Design review of the part shown in the three views and the two pictorial views. Dimensions are in mm from the part's minimum x, y and z. Round coordinates to 2 decimals unless told otherwise and drop trailing zeros. Order: outer loops, then holes, each group sorted by start corner. A loop starts at its lowest first (then second) coordinate and runs counter-clockwise, first axis right, second up.
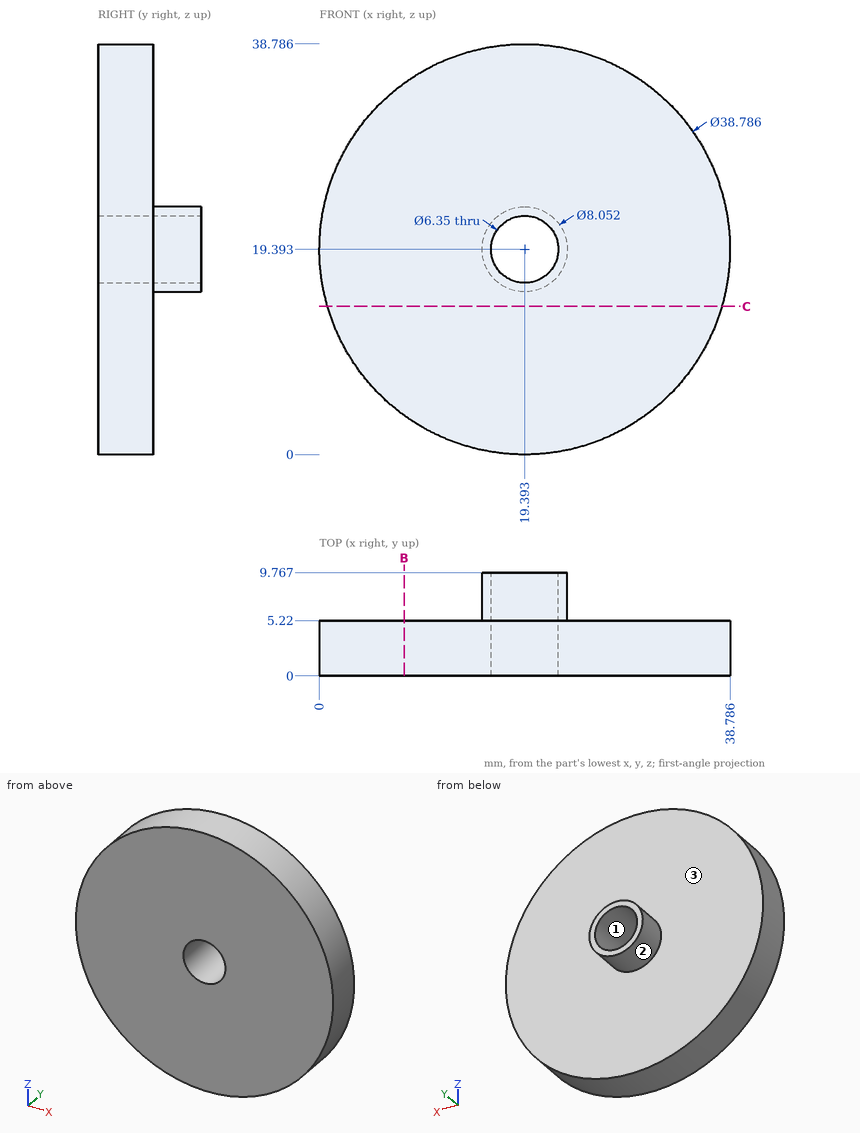
1) Take a section at B-B on x = 8. Give the boundary of the cut face in (y, z).
Results:
outline: (0, 3.7) - (5.22, 3.7) - (5.22, 35.09) - (0, 35.09) - close
2) To check wall thickness, follow line 1 along Y through (x, z) = (31.5, 5); line 2 along Z through (x, y) = (18.5, 2) (1 decimal); line 3 along Z through (x, y) = (12.5, 2.25) (1 decimal). State the ranges of each line that lie inside material, in increasing order.
Results:
line 1: y = 0 to 5.22
line 2: z = 0 to 16.3, 22.4 to 38.8
line 3: z = 1.3 to 37.5
3) Take a section at C-C on z = 14. Give the boundary of the cut face in (x, y) (1 decimal).
Results:
outline: (0.8, 0) - (38, 0) - (38, 5.2) - (0.8, 5.2) - close
4) Clearance check with flat-ended pins moving along their axes: P1, Ø2, axis at y = 8, z = 21, coming from the +X side; P2, Ø1, axis at x = 19, z = 10, coming from the -Y side; P3, Ø3, axis at x = 33.5, y = 6.5, coming from the -Z side (1 decimal); P4, Ø3, axis at x = 8, y = 4.5, coming from the -Z side. State where each tip first meets the part, or that it passes through.
Results:
P1: stops at x = 23.37
P2: stops at y = 0
P3: stops at z = 5.3
P4: stops at z = 2.71
5) The part is to be moulded in two halves that separate along Z. For the marked faces 1, 2 and 3, say which applies: released by +Z, released by -Z, zero draft, split by the parting line, or undercut.
Results:
face 1: undercut
face 2: split by the parting line
face 3: zero draft
